Can you work these out from the drawing? Everything is in mm from the part's minimum corner. Coordinates: 2 decimals unless noted, no trailing zeros. Order: outer loops, then holes, each group sorted by start corner. A loop starts at its lowest first (then second) coordinate and runs counter-clockwise, first axis right, second up. Notation, with made-up numbers: (10.5, 76) -> (29.5, 76) arc R21 cw to (29.5, 91) -> close; hole circle Ø1 at (4.5, 5). An arc over 180 degrees is marked (long way). Put each result on its own line as item: value. Start each with the question number.
Q1. If we section it at B-B (y = 2): Count the separate pieces of the cut face and the enclosed holes in it, and give its area (3 significant figures).
Q2. Please list where these lines run through material, in increasing order: line 1 along Z through (x, y) = (105, 5.5); line 2 along Z through (x, y) = (72, 5.75).
Q3. If we section it at C-C (x = 45): Please give me the cut outline in (y, z), and give its area (3 significant figures).
Q4. Will this pin go through, and if not, where does the flat tip stop? pin 1 (13 mm diameter, centred on x = 45, z = 15, fed in from -Y).
Q5. If we section it at A-A (z = 15): Please give me the cut outline in (x, y), and give its area (3 significant figures).
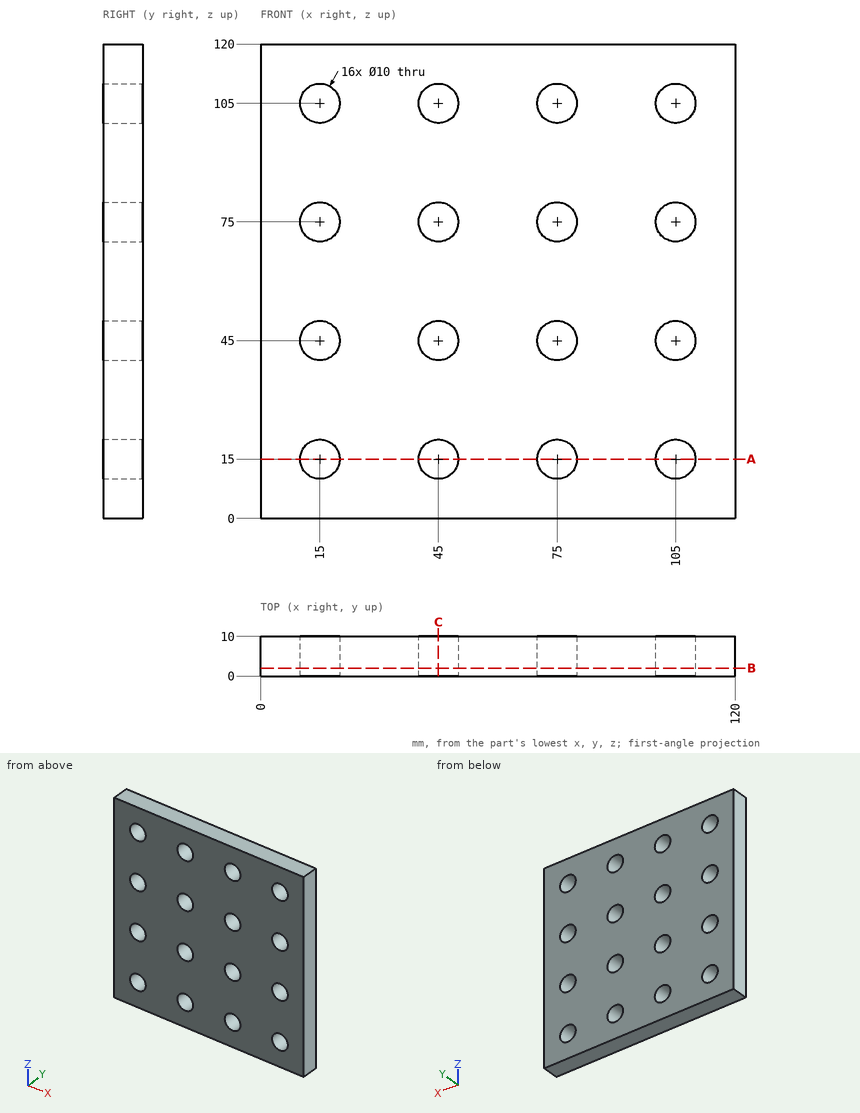
The answers:
1. separate pieces: 1
1. enclosed holes: 16
1. area: 13,100 mm^2
2. line 1: 0 to 10, 20 to 40, 50 to 70, 80 to 100, 110 to 120
2. line 2: 0 to 11, 19 to 41, 49 to 71, 79 to 101, 109 to 120
3. outline: (0, 0) -> (10, 0) -> (10, 10) -> (0, 10) -> close; (0, 20) -> (10, 20) -> (10, 40) -> (0, 40) -> close; (0, 50) -> (10, 50) -> (10, 70) -> (0, 70) -> close; (0, 80) -> (10, 80) -> (10, 100) -> (0, 100) -> close; (0, 110) -> (10, 110) -> (10, 120) -> (0, 120) -> close
3. area: 800 mm^2
4. pin 1: y = 0
5. outline: (0, 0) -> (10, 0) -> (10, 10) -> (0, 10) -> close; (20, 0) -> (40, 0) -> (40, 10) -> (20, 10) -> close; (50, 0) -> (70, 0) -> (70, 10) -> (50, 10) -> close; (80, 0) -> (100, 0) -> (100, 10) -> (80, 10) -> close; (110, 0) -> (120, 0) -> (120, 10) -> (110, 10) -> close
5. area: 800 mm^2
